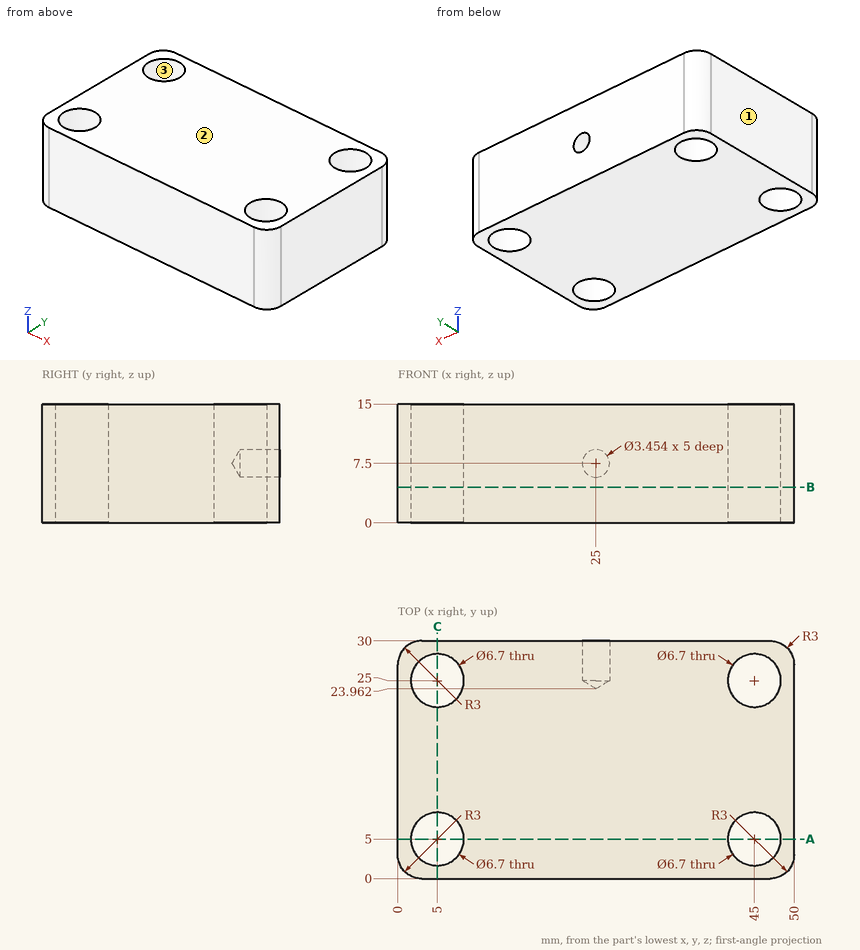
Here's the drawing with two shaded views (mm, measured from the low corner). I have some questions. Give positions to 0.01 mm unless a question says otherwise; leave off trailing zeros. Write each loop counter-clockwise with the first axis right and the second up, starting at its lowest first coordinate (ties: lowest second). Pieces come first, ordered by that corner, then holes. Notation, with made-up numbers: (44.25, -30) -> (73.25, -30) arc R19 cw to (73.25, -26) -> close; hole circle Ø8 at (69, 6). An arc over 180 degrees is marked (long way). Answer as a JSON object with one key per item and string values. Group by question number.
Item 1: We'd pull the mould along X, two halves only. Please class the marked faces 1, 2 and 3: +X half, -X half, draft (parallel to the pull), parting line (faces both ways), or undercut.
Item 2: Suppose I cut it at B-B (z = 4.5). Please give me the cut outline in (x, y).
Item 3: I'm going to push a flat-ended pin straight in: P1, Ø3, axis at x = 25, z = 7.5, coming from the +Y side. Where does the tip first touch, or does it pass through?
Item 4: Suppose I cut it at A-A (y = 5). Please give me the cut outline in (x, z), plus the area to 3 significant figures.
Item 5: Please list where these lines run through material, in increasing order: line 1 (Y direction, x = 45, z = 7.5); line 2 (X direction, y = 6.75, z = 14.75) (1 decimal); line 3 (X direction, y = 26.3, z = 7.5). Write a range as [from, to].
Item 6: Suppose I cut it at C-C (x = 5). Please give me the cut outline in (y, z).
Findings:
{
 "1": {"face 1": "-X half", "face 2": "draft", "face 3": "undercut"},
 "2": {"outline": "(0, 3) arc R3 ccw to (3, 0) -> (47, 0) arc R3 ccw to (50, 3) -> (50, 27) arc R3 ccw to (47, 30) -> (3, 30) arc R3 ccw to (0, 27) -> close; hole circle Ø6.7 at (5, 5); hole circle Ø6.7 at (5, 25); hole circle Ø6.7 at (45, 5); hole circle Ø6.7 at (45, 25)"},
 "3": {"P1": "stops at y = 24.86"},
 "4": {"outline": "(0, 0) -> (1.65, 0) -> (1.65, 15) -> (0, 15) -> close; (8.35, 0) -> (41.65, 0) -> (41.65, 15) -> (8.35, 15) -> close; (48.35, 0) -> (50, 0) -> (50, 15) -> (48.35, 15) -> close", "area": "549 mm²"},
 "5": {"line 1": "y = [0, 1.65], [8.35, 21.65], [28.35, 30]", "line 2": "x = [0, 2.1], [7.9, 42.1], [47.9, 50]", "line 3": "x = [0, 1.91], [8.09, 23.27], [26.73, 41.91], [48.09, 50]"},
 "6": {"outline": "(0, 0) -> (1.65, 0) -> (1.65, 15) -> (0, 15) -> close; (8.35, 0) -> (21.65, 0) -> (21.65, 15) -> (8.35, 15) -> close; (28.35, 0) -> (30, 0) -> (30, 15) -> (28.35, 15) -> close"}
}
